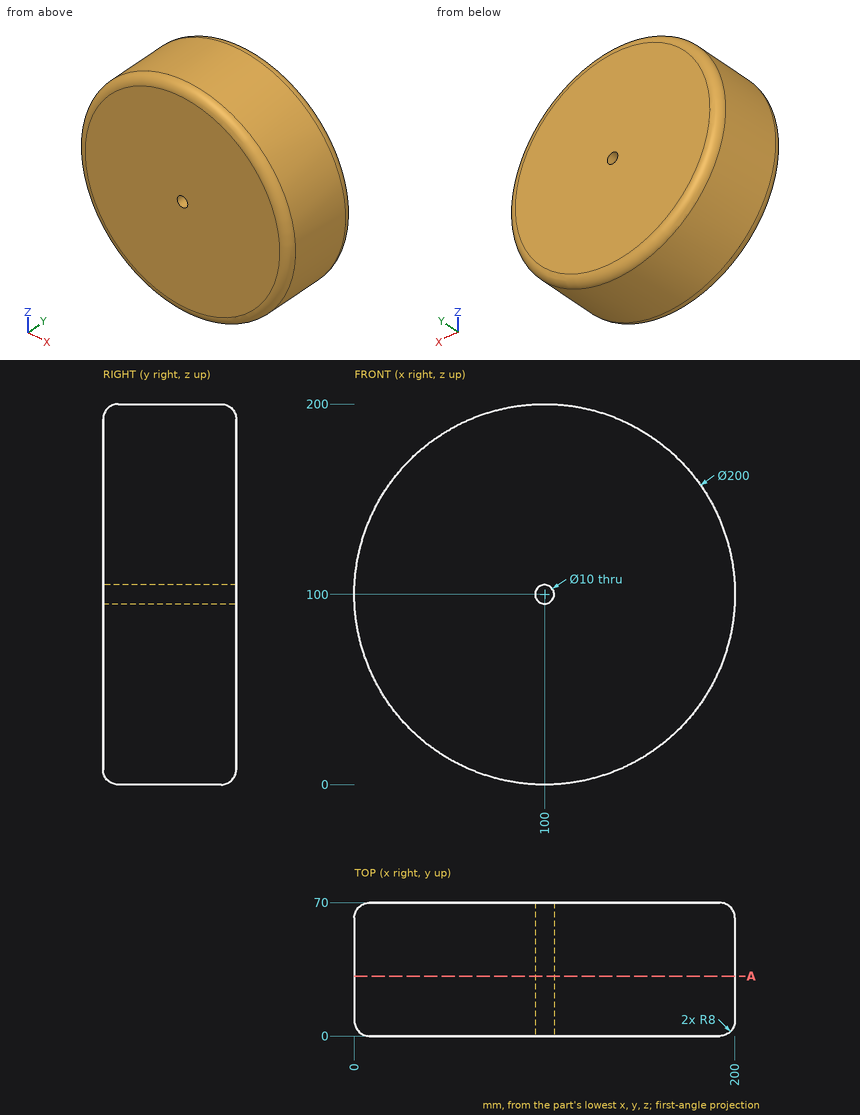
Could you check a few things on this drawing? It's one solid part, dimensions in mm from its lowest x, y, z. Round coordinates to 2 decimals unless told otherwise and drop trailing zeros. Order: outer loops, then holes, each group sorted by start corner. A loop starts at its lowest first (then second) coordinate and runs counter-clockwise, first axis right, second up. Notation, with made-up numbers: M 46,25 L 77,25 A26 cw 77,43 Z; hole C -6.75,64.25 d9. An arc over 180 degrees is marked long. One line per item, written item: value.
(1) Imagine slicing it at A-A (y = 31.5). Write out the boundary of the cut face in (x, z), and give its area (3 significant figures).
Ans:
outline: C 100,100 d200; hole C 100,100 d10
area: 31,300 mm^2
(2) I'm going to push flat-ended pins straight in: P1, Ø13, axis at x = 100, z = 100, coming from the -Y side; P2, Ø8, axis at x = 165.5, z = 175.5, coming from the -Y side; P3, Ø2, axis at y = 27.5, z = 176.5, coming from the +X side; P4, Ø3, axis at y = 33.5, z = 139, coming from the -X side. Where does each tip first touch, or does it pass through?
Ans:
P1: stops at y = 0
P2: stops at y = 1.04
P3: stops at x = 165.57
P4: stops at x = 7.3
(3) I need wall thicknesses on line 1 along X through (y, z) = (53, 100); line 2 along Z through (x, y) = (97, 7); line 3 along Y through (x, z) = (30.5, 34.5). Which ranges of each line are inside material? Lowest first, please. Write a range as from..to.
Ans:
line 1: x = 0..95, 105..200
line 2: z = 0.11..96, 104..199.89
line 3: y = 0.81..69.19
